CAD build for the part. Positions are in the model's coordinates, mm. Face numbers are marked on the shaded views. A direction names the side the tool comes from. Round coordinates to 2 decimals unless told otherwise and drop trailing zeros. Write each loop counter-clockwise with the first axis right and the second up, starting at its lowest first coordinate (ties: lowest second). Pieces come first, ordered by that corner, then holes. Notation, with made-up numbers: (82.5, 54) - (124.5, 54) arc R19 ccw to (124.5, 81) - close; hole circle Ø9 at (11.5, 76). An arc over 180 degrees is marked (long way). Put each result on its own line as item: value. Start each with the question number.
Item 1: Pin check, flat tips, straight feed: pin 1 Ø1.5 at (y, z) = (1, 0.5) entering from +X; pin 2 Ø2 at (y, z) = (1, 2) entering from -X; pin 3 Ø4.5 at (x, y) = (3, -0.5) entering from +Z; pin 4 Ø1.5 at (x, z) = (8, 1.5) entering from -Y. Stop position of each tip, or through.
Item 2: Drill centre lines: line 1 (Y direction, x = 0, z = 0.75) (3 decimals); line 2 (Y direction, x = 5, z = 0.7); line 3 (Z direction, x = -6, y = 9). Where is each one in solid material? Low to high. Write a range as from..to.
Item 3: 3-axis set-ups, long thin cutter, end or side, ignore diameter. For the marked faces 4, 5 and 6: which of +Z, -Z, +X, -X, +Y, -Y reach the whole face in a straight line?
Item 4: Cut at D-D (y = -10.5). Give the cut face in (x, z).
Item 5: Cut at B-B (x = 0). Give the cut face in (y, z) (3 decimals), and give its area (3 significant figures).
Item 6: Cut at A-A (z = 0.8). Count the separate pieces of the cut face and the enclosed holes in it, and give its area (3 significant figures).
Item 7: Cut at C-C (x = 13.5). Give the cut face in (y, z), and give its area (3 significant figures).
Item 8: Mould opens along Y. For the marked faces 1, 2 and 3 say: released by +Y, released by -Y, zero draft, split by the parting line, or undercut.
```python
from build123d import *

# Parameters (mm, degrees)
BOSS_EXTRUDE1_DEPTH   = 3
BOSS_EXTRUDE1_2_DEPTH = 3
BOSS_EXTRUDE1_3_DEPTH = 3
BOSS_EXTRUDE1_4_DEPTH = 3
SKETCH1_R             = 9.45
SKETCH1_R_2           = 7.575
BOSS_EXTRUDE1_5_DEPTH = 3
BOSS_EXTRUDE2_START   = -1
SKETCH2_R             = 15
BOSS_EXTRUDE2_DEPTH   = 1
FILLET1_R             = 0.1
FILLET2_R             = 0.1


with BuildPart() as part:
    # Sketch1 → Boss-Extrude1 (new body)
    with BuildSketch(Plane.XY):
        with BuildLine():
            ThreePointArc((5.814987036, 11.121529831), (6.485587296, 12.198625444), (7.456549067, 13.01537076))
            ThreePointArc((7.456549067, 13.01537076), (0, 15), (-7.456549067, 13.01537076))
            ThreePointArc((-7.456549067, 13.01537076), (-6.485587296, 12.198625444), (-5.814987036, 11.121529831))
            ThreePointArc((-5.814987036, 11.121529831), (0, 12.55), (5.814987036, 11.121529831))
        make_face()
    extrude(amount=BOSS_EXTRUDE1_DEPTH)



with BuildPart() as body_2:
    # Sketch1 → Boss-Extrude1 2 (new body)
    with BuildSketch(Plane.XY):
        with BuildLine():
            ThreePointArc((13.01537076, -7.456549067), (14.495353762, -3.858071967), (15, 0))
            ThreePointArc((15, 0), (14.495353762, 3.858071967), (13.01537076, 7.456549067))
            ThreePointArc((13.01537076, 7.456549067), (12.198625444, 6.485587296), (11.121529831, 5.814987036))
            ThreePointArc((11.121529831, 5.814987036), (12.55, 0), (11.121529831, -5.814987036))
            ThreePointArc((11.121529831, -5.814987036), (12.198625444, -6.485587296), (13.01537076, -7.456549067))
        make_face()
    extrude(amount=BOSS_EXTRUDE1_2_DEPTH)


with BuildPart() as body_3:
    # Sketch1 → Boss-Extrude1 3 (new body)
    with BuildSketch(Plane.XY):
        with BuildLine():
            ThreePointArc((-7.456549067, -13.01537076), (0, -15), (7.456549067, -13.01537076))
            ThreePointArc((7.456549067, -13.01537076), (6.485587296, -12.198625444), (5.814987036, -11.121529831))
            ThreePointArc((5.814987036, -11.121529831), (0, -12.55), (-5.814987036, -11.121529831))
            ThreePointArc((-5.814987036, -11.121529831), (-6.485587296, -12.198625444), (-7.456549067, -13.01537076))
        make_face()
    extrude(amount=BOSS_EXTRUDE1_3_DEPTH)


with BuildPart() as body_4:
    # Sketch1 → Boss-Extrude1 4 (new body)
    with BuildSketch(Plane.XY):
        with BuildLine():
            ThreePointArc((-11.121529831, 5.814987036), (-12.198625444, 6.485587296), (-13.01537076, 7.456549067))
            ThreePointArc((-13.01537076, 7.456549067), (-15, 0), (-13.01537076, -7.456549067))
            ThreePointArc((-13.01537076, -7.456549067), (-12.198625444, -6.485587296), (-11.121529831, -5.814987036))
            ThreePointArc((-11.121529831, -5.814987036), (-12.55, 0), (-11.121529831, 5.814987036))
        make_face()
    extrude(amount=BOSS_EXTRUDE1_4_DEPTH)


with BuildPart() as body_5:
    # Sketch1 → Boss-Extrude1 5 (new body)
    with BuildSketch(Plane.XY):
        Circle(SKETCH1_R)
        Circle(SKETCH1_R_2, mode=Mode.SUBTRACT)
    extrude(amount=BOSS_EXTRUDE1_5_DEPTH)


with BuildPart() as part_1:
    add(part.part)

    add(body_2.part)  # Boss-Extrude2 merges body 2

    add(body_3.part)  # Boss-Extrude2 merges body 3

    add(body_4.part)  # Boss-Extrude2 merges body 4

    add(body_5.part)  # Boss-Extrude2 merges body 5
    # Sketch2 → Boss-Extrude2 (add)
    with BuildSketch(Plane.XY.offset(BOSS_EXTRUDE2_START)):
        with Locations(Location((0, 0, 0), (0, 0, 150.191461703))):
            Circle(SKETCH2_R)
    extrude(amount=BOSS_EXTRUDE2_DEPTH)

    # Fillet1
    fillet1_edges = [part_1.edges().sort_by_distance(p)[0] for p in [
        (11.121529831, 5.814987036, 1.5),
        (11.121529831, -5.814987036, 1.5),
        (5.814987036, -11.121529831, 1.5),
        (-5.814987036, -11.121529831, 1.5),
        (-11.121529831, -5.814987036, 1.5),
        (-11.121529831, 5.814987036, 1.5),
        (5.814987036, 11.121529831, 1.5),
        (-5.814987036, 11.121529831, 1.5),
    ]]
    fillet(fillet1_edges, radius=FILLET1_R)

    # Fillet2
    fillet2_edges = [part_1.edges().sort_by_distance(p)[0] for p in [
        (6.520367717, 12.238227379, 3),
        (12.238227379, -6.520367717, 3),
        (-6.520367717, -12.238227379, 3),
        (-12.238227379, 6.520367717, 3),
        (-9.45, 0, 3),
        (0, -12.55, 3),
        (6.520367717, -12.238227379, 3),
        (5.799143147, -11.164972845, 3),
        (-5.799143147, -11.164972845, 3),
        (12.55, 0, 3),
        (12.238227379, 6.520367717, 3),
        (11.164972845, 5.799143147, 3),
        (11.164972845, -5.799143147, 3),
        (0, 12.55, 3),
        (-6.520367717, 12.238227379, 3),
        (-5.799143147, 11.164972845, 3),
        (5.799143147, 11.164972845, 3),
        (-12.55, 0, 3),
        (-12.238227379, -6.520367717, 3),
        (-11.164972845, -5.799143147, 3),
        (-11.164972845, 5.799143147, 3),
    ]]
    fillet(fillet2_edges, radius=FILLET2_R - 0.0001)  # a hair under: the kernel refuses the full size


solid = part_1.part
```
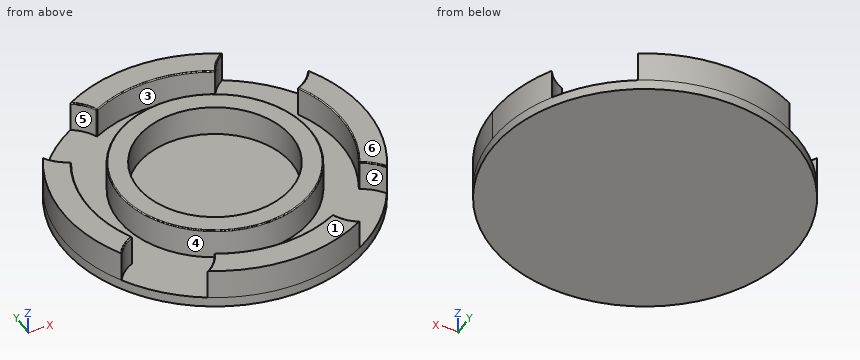
Output values:
1. pin 1: x = 15
1. pin 2: x = -15
1. pin 3: z = 0
1. pin 4: y = -13.13
2. line 1: -15..-12.55, -9.45..-7.575, 7.575..9.45, 12.55..15
2. line 2: -14.14..-11.51, -8.02..-5.69, 5.69..8.02, 11.51..14.14
2. line 3: -1..0
3. face 4: +Z
3. face 5: +Z, -X
3. face 6: +Z, +X, -X, +Y, -Y
4. outline: (-10.71, -1) - (10.71, -1) - (10.71, 0) - (-10.71, 0) - close
5. outline: (-15, -1) - (15, -1) - (15, 3) - (12.65, 3) arc R0.1 ccw to (12.55, 2.9) - (12.55, 0) - (9.45, 0) - (9.45, 2.9) arc R0.1 ccw to (9.35, 3) - (7.575, 3) - (7.575, 0) - (-7.575, 0) - (-7.575, 3) - (-9.35, 3) arc R0.1 ccw to (-9.45, 2.9) - (-9.45, 0) - (-12.55, 0) - (-12.55, 2.9) arc R0.1 ccw to (-12.65, 3) - (-15, 3) - close
5. area: 55.9 mm2
6. separate pieces: 5
6. enclosed holes: 1
6. area: 233 mm2
7. outline: (-6.54, -1) - (6.54, -1) - (6.54, 3) - (-6.54, 3) - close
7. area: 52.3 mm2
8. face 1: zero draft
8. face 2: released by -Y
8. face 3: undercut
